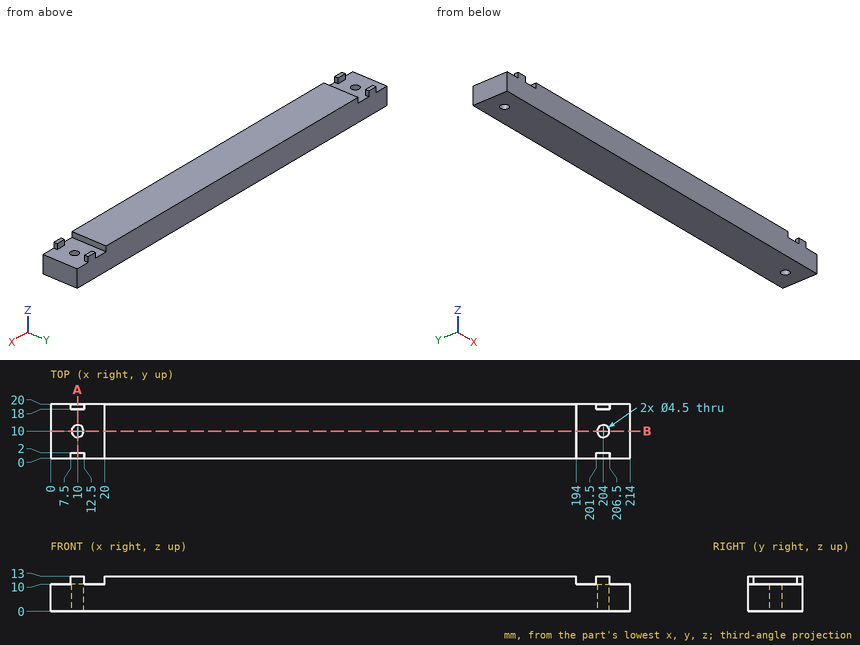
Geometry: see drawing. Coordinates: mm, zero at the bounding-box minimum. Coordinates: 2 decimals unless noted, no trailing zeros. Order: outer loops, then holes, each group sorted by start corner. A loop starts at its lowest first (then second) coordinate and runs counter-clockwise, first axis right, second up. Notation, with made-up numbers: M -31,54 L 26,54 A24 cw 26,80 Z; hole C 2,41 d7. An arc over 180 degrees is marked long. Answer in a Markdown table with one row per item. Add a question column.
Q1. Contact query for flat-ended pins moving along their axis: P1, Ø1.6, axis at y = 1.5, z = 11, coming from the -X side; P2, Ø0.6, axis at y = 1, z = 11, coming from the +X side; P3, Ø1, axis at y = 7.5, z = 11, coming from the -X side; P4, Ø2.5, axis at x = 10, y = 10, coming from the +Z side. Output: stop coordinate, or through.
Q2. Line query: L1, parallel to X at y = 19, z = 12; L2, parallel to Y at x = 204, z = 2.5; L3, parallel to X at y = 13.25, z = 11.25. Output: solid intervals per line, ascending.
Q3. Section query B-B on y = 10. Return the cut outline in (x, z), and give its area (3 significant figures).
Q4. Section query A-A on x = 10. Return the cut outline in (y, z), and give its area (3 significant figures).
Completed:
| question | item | result |
|---|---|---|
| 1 | P1 | stops at x = 7.5 |
| 1 | P2 | stops at x = 206.5 |
| 1 | P3 | stops at x = 20 |
| 1 | P4 | passes through |
| 2 | L1 | x = 7.5 to 12.5, 20 to 194, 201.5 to 206.5 |
| 2 | L2 | y = 0 to 7.75, 12.25 to 20 |
| 2 | L3 | x = 20 to 194 |
| 3 | outline | M 0,0 L 7.75,0 L 7.75,10 L 0,10 Z; M 12.25,0 L 201.75,0 L 201.75,10 L 194,10 L 194,13 L 20,13 L 20,10 L 12.25,10 Z; M 206.25,0 L 214,0 L 214,10 L 206.25,10 Z |
| 3 | area | 2,570 mm2 |
| 4 | outline | M 0,0 L 7.75,0 L 7.75,10 L 2,10 L 2,13 L 0,13 Z; M 12.25,0 L 20,0 L 20,13 L 18,13 L 18,10 L 12.25,10 Z |
| 4 | area | 167 mm2 |
